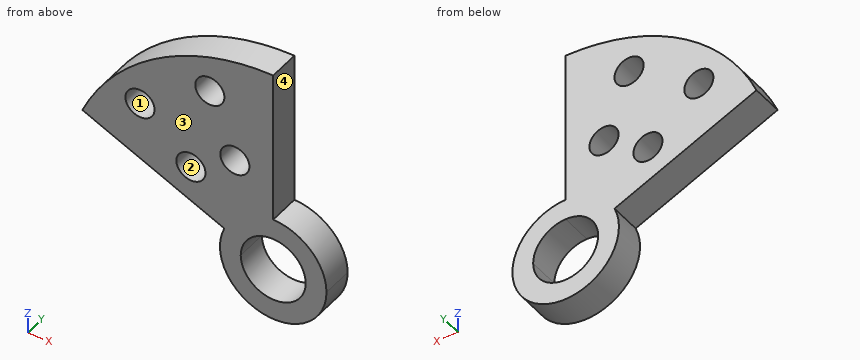
```python
from build123d import *

# Parameters (mm, degrees)
F0_R     = 1.4
F1_DEPTH = 3


# Not quite as in the source:
# - a feature names something its author has since deleted; it is built from what else it names


with BuildPart() as f1:
    # F0 (on Front) → F1 (new body)
    with BuildSketch(Plane.XZ):
        with BuildLine():
            Line((-5.125, 0), (-3.125, 0))
            ThreePointArc((-3.125, 0), (-3.0593081858, 0.6373840479), (-2.8649946083, 1.2479707105))
            Line((-2.8649946083, 1.2479707105), (-4.700755545, 2.0416959387))
            ThreePointArc((-4.700755545, 2.0416959387), (-5.0178181099, 1.0426535455), (-5.125, 0))
        make_face()
        with BuildLine():
            ThreePointArc((3.125, 0), (0, -3.125), (-3.125, 0))
            Line((-3.125, 0), (-5.125, 0))
            ThreePointArc((-5.125, 0), (0, -5.125), (5.125, 0))
            ThreePointArc((5.125, 0), (3.6239222536, 3.6239222536), (0, 5.125))
            Line((0, 5.125), (0, 3.125))
            ThreePointArc((0, 3.125), (2.2097086912, 2.2097086912), (3.125, 0))
        make_face()
        with BuildLine():
            Line((-4.700755545, 2.0416959387), (-2.8649946083, 1.2479707105))
            ThreePointArc((-2.8649946083, 1.2479707105), (-1.7125589814, 2.6139561464), (0, 3.125))
            Line((0, 3.125), (0, 5.125))
            ThreePointArc((0, 5.125), (-2.8108658198, 4.2854006047), (-4.700755545, 2.0416959387))
        make_face()
        with BuildLine():
            Line((-18.3542016569, 7.9450161447), (-4.700755545, 2.0416959387))
            ThreePointArc((-4.700755545, 2.0416959387), (-2.8108658198, 4.2854006047), (0, 5.125))
            Line((0, 5.125), (0, 20))
            ThreePointArc((0, 20), (-10.9795190493, 16.7167628878), (-18.3542016569, 7.9450161447))
        make_face()
        with Locations((-7.9143406, 6.9087709696)):
            Circle(F0_R, mode=Mode.SUBTRACT)
        with Locations((-3.6882084925, 9.5327961412)):
            Circle(F0_R, mode=Mode.SUBTRACT)
        with Locations((-12.8110766731, 11.1833441447)):
            Circle(F0_R, mode=Mode.SUBTRACT)
        with Locations((-6.0959799545, 15.5703980315)):
            Circle(F0_R, mode=Mode.SUBTRACT)
    extrude(amount=F1_DEPTH)


solid = f1.part
```
Input: part model. Units: mm. Frame: model coordinates. Face numbers are marked on the shaded views. Give positions to 0.01 mm unless a question says otherwise; leave off trailing zeros. Write each loop counter-clockwise with the first axis right and the second up, starting at its lowest first coordinate (ties: lowest second). Pieces come first, ordered by that corner, then holes. Notation, with made-up numbers: (68, 35) - (86, 35) arc R27 cw to (86, 56) - close; hole circle Ø4 at (-9, 59). An arc over 180 degrees is marked (long way). Write item = value, one per line. Start each with the question number.
1. Mould query, pull axis X, two halves, no side actions, for the marked faces 1, 2, 3 and 4. Classes: released by +X, released by -X, zero draft, split by the parting line, or undercut.
2. Section query A-A, the plane x = -6. Output: boundary loops of the cut face in (y, z), then the cut area to 3 significant figures.
3. Section query C-C, the plane x = -9. Output: boundary loops of the cut face in (y, z).
4. Section query D-D, the plane x = -16. Output: boundary loops of the cut face in (y, z).
5. Ray query, L1, parallel to X at y = -1.9, z = 10; L2, parallel to X at y = -0.8, z = 10.75; L3, parallel to X at y = -1.3, z = 8.75. Return the intervals inside material, ascending.
6. First-contact query: pin 1 Ø1.5 at (y, z) = (-2, 10.5) entering from -X; pin 2 Ø1.5 at (x, y) = (-11.5, -2.5) entering from -Z; pin 3 Ø1.5 at (x, y) = (-11.5, -2.5) entering from +Z. Flat tips, straight axial feed; report the tip coordinate or a pass-through.
7. Section query B-B, the plane y = -2.55. Output: boundary loops of the cut face in (x, z) (3 decimals).
Check sheet entries:
q1.face_1 = undercut
q1.face_2 = undercut
q1.face_3 = zero draft
q1.face_4 = released by +X
q2.outline = (-3, 2.6) - (0, 2.6) - (0, 14.17) - (-3, 14.17) - close; (-3, 16.97) - (0, 16.97) - (0, 19.08) - (-3, 19.08) - close
q2.area = 41.0 mm2
q3.outline = (-3, 3.9) - (0, 3.9) - (0, 6.02) - (-3, 6.02) - close; (-3, 7.79) - (0, 7.79) - (0, 17.86) - (-3, 17.86) - close
q4.outline = (-3, 6.93) - (0, 6.93) - (0, 12) - (-3, 12) - close
q5.L1 = -17.32 to -13.56, -12.06 to -5.01, -2.37 to 0
q5.L2 = -16.87 to -14.14, -11.48 to -4.38, -3 to 0
q5.L3 = -17.98 to -4.85, -2.53 to 0
q6.pin_1 = -17.46
q6.pin_2 = 4.66
q6.pin_3 = 16.87
q7.outline = (-18.354, 7.945) - (-4.701, 2.042) arc R5.125 ccw (long way) to (0, 5.125) - (0, 20) arc R20 ccw to start; hole circle Ø2.8 at (-12.811, 11.183); hole circle Ø2.8 at (-7.914, 6.909); hole circle Ø2.8 at (-6.096, 15.57); hole circle Ø2.8 at (-3.688, 9.533); hole circle Ø6.25 at (0, 0)
